Read the model definition and answer for the solid it produces. Units are mm, in the model's axes. A direction names the side the tool comes from. Give positions to 0.01 mm unless a question says otherwise; leave off trailing zeros. Order: outer loops, then holes, each group sorted by start corner. A loop starts at its lowest first (then second) coordinate and runs counter-clockwise, first axis right, second up. Notation, with made-up numbers: (-39.5, 35) - (-33.5, 35) arc R20 cw to (-33.5, 64) - close; hole circle Ø3 at (-12, 64). An arc over 180 degrees is marked (long way). Write each question's results on one line, items separated by ' | '.
from build123d import *

# Parameters (mm, degrees)
F1_DEPTH = 25


with BuildPart() as f1:
    # F0 (on Front) → F1 (new body)
    with BuildSketch(Plane.XZ):
        with BuildLine():
            Line((5, 0), (0, 0))
            Line((0, 0), (0, -19.23344))
            ThreePointArc((0, -19.23344), (7.5, -40), (0, -60.76656))
            Line((0, -60.76656), (0, -85))
            Line((0, -85), (5, -85))
            Line((5, -85), (5, -62.5))
            ThreePointArc((5, -62.5), (12.5, -40), (5, -17.5))
            Line((5, -17.5), (5, 0))
        make_face()
    extrude(amount=F1_DEPTH)


solid = f1.part
(1) Section A-A (x = 1.5) is taken. Give the vertices of the cut face in (y, z), plus the area to 3 significant figures.
Conclusion:
outline: (-25, -85) - (0, -85) - (0, -58.81) - (-25, -58.81) - close; (-25, -21.19) - (0, -21.19) - (0, 0) - (-25, 0) - close | area: 1,180 mm^2
(2) The mould has two halves that part along Z. Classify faces 4 (the face through (12.5, -12.3, -40.3)), 5 (the face through (0, -12, -73)), 6 (the face through (7.5, -12.3, -39.7)): pulls with the +Z half, pulls with the -Z half, needs draft (parallel to the pull), parting line crosses it, or undercut.
Conclusion:
face 4: parting line crosses it | face 5: needs draft | face 6: undercut
(3) Section B-B (y = -6.75) is taken. Give the vertices of the cut face in (x, z), plus the area to 3 significant figures.
Conclusion:
outline: (0, -85) - (5, -85) - (5, -62.5) arc R37.5 ccw to (5, -17.5) - (5, 0) - (0, 0) - (0, -19.23) arc R32.5 cw to (0, -60.77) - close | area: 442 mm^2
(4) Section D-D (x = 10.25) is taken. Give the vertices of the cut face in (y, z).
Conclusion:
outline: (-25, -52.79) - (0, -52.79) - (0, -27.21) - (-25, -27.21) - close
(5) Each of these flat-tipped pins is pushed along its axis until it touches: pin 1 (3 mm diameter, centred on y = -22, z = -33, fed in from -X); pin 2 (1.5 mm diameter, centred on x = 4.5, y = -14.5, fed in from +Z); pin 3 (2 mm diameter, centred on x = 10.5, y = -17.5, fed in from -Z); pin 4 (1.5 mm diameter, centred on x = 10.5, y = -5.5, fed in from -Z). Where does it stop, or does it pass through?
Conclusion:
pin 1: x = 6.37 | pin 2: z = 0 | pin 3: z = -54.7 | pin 4: z = -54.1
(6) For faces 1 (the face through (3, -12, 0)), 2 (the face through (5, -12, -9)), 3 (the face through (5, -12, -74)), determine the directions among +Z, -Z, +X, -X, +Y, -Y from which every point of the face is accessible in a straight line to the end or side of a thin tool.
Conclusion:
face 1: +Z, +X, -X, +Y, -Y | face 2: +Z, +X, +Y, -Y | face 3: -Z, +X, +Y, -Y
(7) Section C-C (z = -44) is taken. Give the vertices of the cut face in (x, y).
Conclusion:
outline: (7.25, -25) - (12.29, -25) - (12.29, 0) - (7.25, 0) - close
(8) Consider probe 1 along X at (y, z) = (-3.5, -68.5); probe 2 along Z at (x, y) = (0.5, -10.25); probe 3 along Z at (x, y) = (1.25, -9). Determine where each line is inside the solid, lowest interval first. Write a range as [from, to].
Conclusion:
probe 1: [0, 5] | probe 2: [-85, -60.15], [-19.85, 0] | probe 3: [-85, -59.16], [-20.84, 0]
